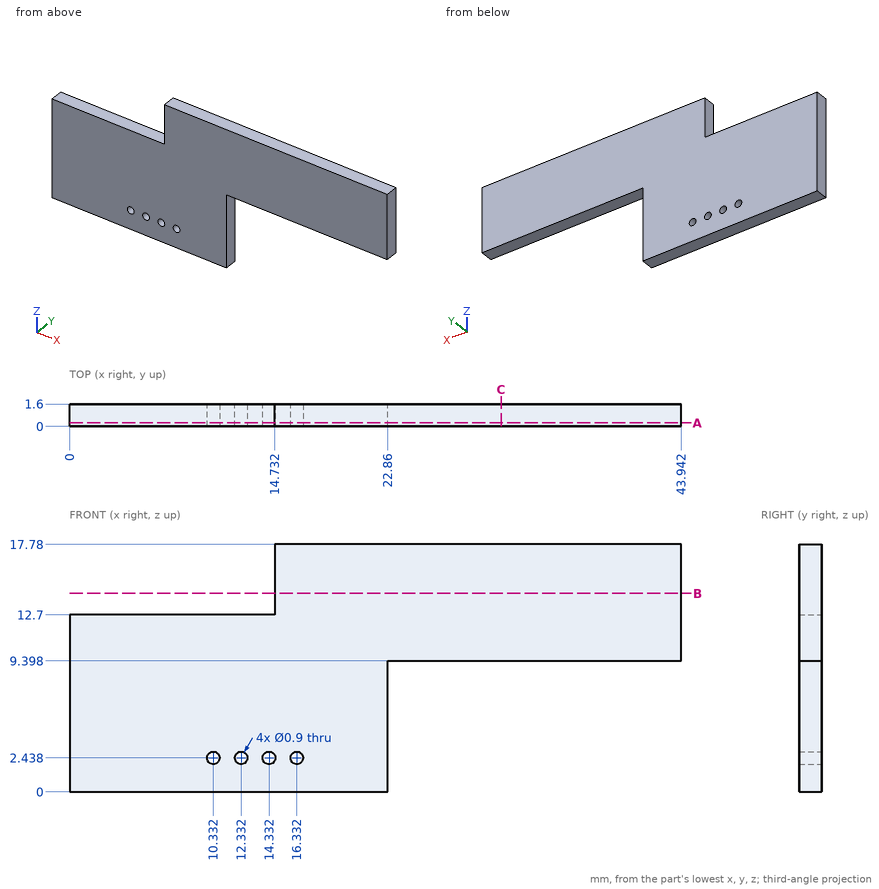
Design review of the part shown in the three views and the two pictorial views. Dimensions are in mm from the part's minimum x, y and z. Give positions to 0.01 mm unless a question says otherwise; leave off trailing zeros. Loops run counter-clockwise (first coordinate to the right, second up) from the corner with the lowest first, then second, coordinate; pieces in that order, holes last. Notation, with made-up numbers: (81, 12) -> (135, 12) arc R18 ccw to (135, 47) -> close; hole circle Ø4 at (6.25, 40.25). An arc over 180 degrees is marked (long way). One line per item, written item: value.
Q1. We need section B-B on z = 14.25. Give the boundary of the cut face in (x, y).
Numbers:
outline: (14.73, 0) -> (43.94, 0) -> (43.94, 1.6) -> (14.73, 1.6) -> close
Q2. For pin 1 Ø0.8 at (y, z) = (1, 3) entering from +X; pin 2 Ø0.8 at (y, z) = (1, 14.5) entering from -X; pin 3 Ø0.8 at (x, y) = (33, 1) entering from -Z, all flat-tipped, find the tip position at first contact; note any pin that passes through.
Numbers:
pin 1: stops at x = 22.86
pin 2: stops at x = 14.73
pin 3: stops at z = 9.4
Q3. For L1, parallel to Z at x = 39, y = 1.4; L2, parallel to X at y = 0.95, z = 6; L3, parallel to X at y = 1.25, z = 15.75, list the stretches that pass through material, from the lowest coordinate up.
Numbers:
L1: z = 9.4 to 17.78
L2: x = 0 to 22.86
L3: x = 14.73 to 43.94
Q4. We need section A-A on y = 0.25. Give the boundary of the cut face in (x, z).
Numbers:
outline: (0, 0) -> (22.86, 0) -> (22.86, 9.4) -> (43.94, 9.4) -> (43.94, 17.78) -> (14.73, 17.78) -> (14.73, 12.7) -> (0, 12.7) -> close; hole circle Ø0.9 at (10.33, 2.44); hole circle Ø0.9 at (12.33, 2.44); hole circle Ø0.9 at (14.33, 2.44); hole circle Ø0.9 at (16.33, 2.44)
Q5. We need section C-C on x = 31. Give the boundary of the cut face in (y, z).
Numbers:
outline: (0, 9.4) -> (1.6, 9.4) -> (1.6, 17.78) -> (0, 17.78) -> close
